Drawing for the job (mm, zero at the part's lowest x, y, z). Give positions to 0.01 mm unless a question says otherwise; leave off trailing zeros. Order: outer loops, then holes, each group sorted by start corner. A loop starts at its lowest first (then second) coordinate and runs counter-clockwise, first axis right, second up. Notation, with made-up numbers: (33, 67) - (70, 67) arc R23 cw to (70, 98) - close; hole circle Ø7 at (68.5, 43.25). An arc over 180 degrees is marked (long way). One line per item, written item: value.
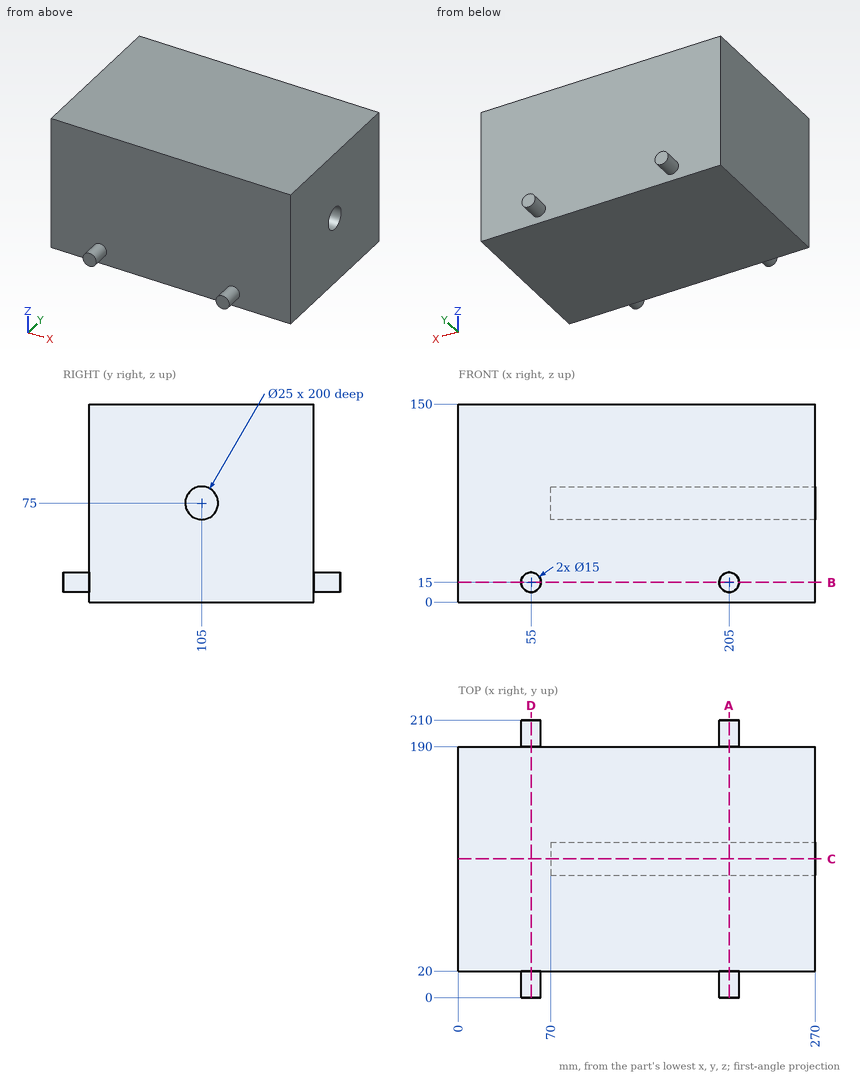
(1) Slice it at C-C, the plane y = 105. Give the cut face in (x, z).
Completed:
outline: (0, 0) - (270, 0) - (270, 62.5) - (70, 62.5) - (70, 87.5) - (270, 87.5) - (270, 150) - (0, 150) - close
(2) Pin check, flat tips, straight feed: P1, Ø1, axis at x = 53.5, z = 124, coming from the +Y side; P2, Ø10, axis at x = 199.5, z = 49.5, coming from the -Y side. Stop position of each tip, or through.
Completed:
P1: y = 190
P2: y = 20
(3) Slice it at D-D, the plane x = 55. Give the cut face in (y, z).
Completed:
outline: (0, 7.5) - (20, 7.5) - (20, 0) - (190, 0) - (190, 7.5) - (210, 7.5) - (210, 22.5) - (190, 22.5) - (190, 150) - (20, 150) - (20, 22.5) - (0, 22.5) - close
(4) Slice it at B-B, the plane z = 15. Give the cut face in (x, y).
Completed:
outline: (0, 20) - (47.5, 20) - (47.5, 0) - (62.5, 0) - (62.5, 20) - (197.5, 20) - (197.5, 0) - (212.5, 0) - (212.5, 20) - (270, 20) - (270, 190) - (212.5, 190) - (212.5, 210) - (197.5, 210) - (197.5, 190) - (62.5, 190) - (62.5, 210) - (47.5, 210) - (47.5, 190) - (0, 190) - close
(5) Slice it at A-A, the plane x = 205. Give the cut face in (y, z), and give its area (3 significant figures).
Completed:
outline: (0, 7.5) - (20, 7.5) - (20, 0) - (190, 0) - (190, 7.5) - (210, 7.5) - (210, 22.5) - (190, 22.5) - (190, 150) - (20, 150) - (20, 22.5) - (0, 22.5) - close; hole circle Ø25 at (105, 75)
area: 25,600 mm²
(6) Drill centre lines: line 1 (Y direction, x = 187, z = 75); line 2 (Y direction, x = 239, z = 133.5); line 3 (Z direction, x = 231.5, y = 108). Where is each one in solid material? Low to high.
Completed:
line 1: 20 to 92.5, 117.5 to 190
line 2: 20 to 190
line 3: 0 to 62.87, 87.13 to 150
